from build123d import *

# Parameters (mm, degrees)
SKETCH1_W           = 55
SKETCH1_H           = 80
BOSS_EXTRUDE1_DEPTH = 10
BOSS_EXTRUDE2_DEPTH = 20
BOSS_EXTRUDE3_DEPTH = 30
FILLET1_START       = -1
FILLET1_DEPTH       = 12


with BuildPart() as part:
    # Sketch1 → Boss-Extrude1 (new body)
    # profile 1 of 11: a face of its own
    with BuildSketch(Plane(origin=(0, 0, 0), x_dir=(1, 0, 0), z_dir=(0, 1, 0))):
        with BuildLine():
            ThreePointArc((-40, 70), (-60, 50), (-40, 30))
            Line((-40, 30), (-40, 40))
            ThreePointArc((-40, 40), (-47.071067812, 57.071067812), (-30, 50))
            Line((-30, 50), (-20, 50))
            ThreePointArc((-20, 50), (-25.857864376, 64.142135624), (-40, 70))
        make_face()
    # profile 2 of 11: a face of its own
    with BuildSketch(Plane(origin=(0, 0, 0), x_dir=(1, 0, 0), z_dir=(0, 1, 0))):
        with BuildLine():
            Line((-40, 40), (-40, 30))
            ThreePointArc((-40, 30), (-25.857864376, 35.857864376), (-20, 50))
            Line((-20, 50), (-30, 50))
            ThreePointArc((-30, 50), (-32.928932188, 42.928932188), (-40, 40))
        make_face()
    # profile 3 of 11: a face of its own
    with BuildSketch(Plane(origin=(0, 0, 0), x_dir=(1, 0, 0), z_dir=(0, 1, 0))):
        with BuildLine():
            ThreePointArc((-40, 70), (-60, 50), (-40, 30))
            Line((-40, 30), (-40, 40))
            ThreePointArc((-40, 40), (-47.071067812, 57.071067812), (-30, 50))
            Line((-30, 50), (-20, 50))
            ThreePointArc((-20, 50), (-25.857864376, 64.142135624), (-40, 70))
        make_face()
    # profile 4 of 11: a face of its own
    with BuildSketch(Plane(origin=(0, 0, 0), x_dir=(1, 0, 0), z_dir=(0, 1, 0))):
        with BuildLine():
            Line((-40, 40), (-40, 30))
            ThreePointArc((-40, 30), (-25.857864376, 35.857864376), (-20, 50))
            Line((-20, 50), (-30, 50))
            ThreePointArc((-30, 50), (-32.928932188, 42.928932188), (-40, 40))
        make_face()
    # profile 5 of 11: a face of its own
    with BuildSketch(Plane(origin=(0, 0, 0), x_dir=(1, 0, 0), z_dir=(0, 1, 0))):
        with BuildLine():
            ThreePointArc((-20, 50), (-25.857864376, 35.857864376), (-40, 30))
            Line((-40, 30), (-27.5, 30))
            Line((-27.5, 30), (27.5, 30))
            Line((27.5, 30), (40, 30))
            ThreePointArc((40, 30), (25.857864376, 35.857864376), (20, 50))
            Line((20, 50), (-20, 50))
        make_face()
    # profile 6 of 11: a face of its own
    with BuildSketch(Plane(origin=(0, 0, 0), x_dir=(1, 0, 0), z_dir=(0, 1, 0))):
        with BuildLine():
            ThreePointArc((60, 50), (54.142135624, 64.142135624), (40, 70))
            ThreePointArc((40, 70), (25.857864376, 64.142135624), (20, 50))
            Line((20, 50), (30, 50))
            ThreePointArc((30, 50), (40, 60), (50, 50))
            ThreePointArc((50, 50), (47.071067812, 42.928932188), (40, 40))
            Line((40, 40), (40, 30))
            ThreePointArc((40, 30), (54.142135624, 35.857864376), (60, 50))
        make_face()
    # profile 7 of 11: a face of its own
    with BuildSketch(Plane(origin=(0, 0, 0), x_dir=(1, 0, 0), z_dir=(0, 1, 0))):
        with BuildLine():
            Line((30, 50), (20, 50))
            ThreePointArc((20, 50), (25.857864376, 35.857864376), (40, 30))
            Line((40, 30), (40, 40))
            ThreePointArc((40, 40), (32.928932188, 42.928932188), (30, 50))
        make_face()
    # profile 8 of 11: a face of its own
    with BuildSketch(Plane(origin=(0, 0, 0), x_dir=(1, 0, 0), z_dir=(0, 1, 0))):
        with BuildLine():
            ThreePointArc((60, 50), (54.142135624, 64.142135624), (40, 70))
            ThreePointArc((40, 70), (25.857864376, 64.142135624), (20, 50))
            Line((20, 50), (30, 50))
            ThreePointArc((30, 50), (40, 60), (50, 50))
            ThreePointArc((50, 50), (47.071067812, 42.928932188), (40, 40))
            Line((40, 40), (40, 30))
            ThreePointArc((40, 30), (54.142135624, 35.857864376), (60, 50))
        make_face()
    # profile 9 of 11: a face of its own
    with BuildSketch(Plane(origin=(0, 0, 0), x_dir=(1, 0, 0), z_dir=(0, 1, 0))):
        with BuildLine():
            Line((30, 50), (20, 50))
            ThreePointArc((20, 50), (25.857864376, 35.857864376), (40, 30))
            Line((40, 30), (40, 40))
            ThreePointArc((40, 40), (32.928932188, 42.928932188), (30, 50))
        make_face()
    # profile 10 of 11: a face of its own
    with BuildSketch(Plane(origin=(0, 0, 0), x_dir=(1, 0, 0), z_dir=(0, 1, 0))):
        with Locations((0, -10)):
            Rectangle(SKETCH1_W, SKETCH1_H)
        with BuildLine():
            ThreePointArc((-7.5, -36.09420366), (-17.5, -26.09420366), (-7.5, -16.09420366))
            Line((-7.5, -16.09420366), (7.5, -16.09420366))
            ThreePointArc((7.5, -16.09420366), (17.5, -26.09420366), (7.5, -36.09420366))
            Line((7.5, -36.09420366), (-7.5, -36.09420366))
        make_face(mode=Mode.SUBTRACT)
    # profile 11 of 11: a face of its own
    with BuildSketch(Plane(origin=(0, 0, 0), x_dir=(1, 0, 0), z_dir=(0, 1, 0))):
        with BuildLine():
            Line((40, 70), (-40, 70))
            ThreePointArc((-40, 70), (-25.857864376, 64.142135624), (-20, 50))
            Line((-20, 50), (20, 50))
            ThreePointArc((20, 50), (25.857864376, 64.142135624), (40, 70))
        make_face()
    extrude(amount=BOSS_EXTRUDE1_DEPTH)

    # Sketch2 → Boss-Extrude2 (add)
    with BuildSketch(Plane(origin=(0, 10, 0), x_dir=(1, 0, 0), z_dir=(0, 1, 0))):
        with BuildLine():
            ThreePointArc((40, 30), (30, 32.679491924), (22.679491924, 40))
            Line((22.679491924, 40), (-22.679491924, 40))
            ThreePointArc((-22.679491924, 40), (-30, 32.679491924), (-40, 30))
            Line((-40, 30), (-27.5, 30))
            Line((-27.5, 30), (27.5, 30))
            Line((27.5, 30), (40, 30))
        make_face()
        with BuildLine():
            ThreePointArc((50, 50), (47.071067812, 42.928932188), (40, 40))
            Line((40, 40), (22.679491924, 40))
            ThreePointArc((22.679491924, 40), (30, 32.679491924), (40, 30))
            ThreePointArc((40, 30), (54.142135624, 35.857864376), (60, 50))
            ThreePointArc((60, 50), (54.142135624, 64.142135624), (40, 70))
            ThreePointArc((40, 70), (30, 67.320508076), (22.679491924, 60))
            Line((22.679491924, 60), (40, 60))
            ThreePointArc((40, 60), (47.071067812, 57.071067812), (50, 50))
        make_face()
        with BuildLine():
            Line((22.679491924, 40), (40, 40))
            ThreePointArc((40, 40), (30, 50), (40, 60))
            Line((40, 60), (22.679491924, 60))
            ThreePointArc((22.679491924, 60), (20, 50), (22.679491924, 40))
        make_face()
        with BuildLine():
            ThreePointArc((50, 50), (47.071067812, 42.928932188), (40, 40))
            Line((40, 40), (22.679491924, 40))
            ThreePointArc((22.679491924, 40), (30, 32.679491924), (40, 30))
            ThreePointArc((40, 30), (54.142135624, 35.857864376), (60, 50))
            ThreePointArc((60, 50), (54.142135624, 64.142135624), (40, 70))
            ThreePointArc((40, 70), (30, 67.320508076), (22.679491924, 60))
            Line((22.679491924, 60), (40, 60))
            ThreePointArc((40, 60), (47.071067812, 57.071067812), (50, 50))
        make_face()
        with BuildLine():
            ThreePointArc((-40, 30), (-30, 32.679491924), (-22.679491924, 40))
            Line((-22.679491924, 40), (-40, 40))
            ThreePointArc((-40, 40), (-50, 50), (-40, 60))
            Line((-40, 60), (-22.679491924, 60))
            ThreePointArc((-22.679491924, 60), (-30, 67.320508076), (-40, 70))
            ThreePointArc((-40, 70), (-60, 50), (-40, 30))
        make_face()
        with BuildLine():
            Line((-40, 40), (-22.679491924, 40))
            ThreePointArc((-22.679491924, 40), (-20.681483474, 44.823619098), (-20, 50))
            ThreePointArc((-20, 50), (-20.681483474, 55.176380902), (-22.679491924, 60))
            Line((-22.679491924, 60), (-40, 60))
            ThreePointArc((-40, 60), (-32.928932188, 57.071067812), (-30, 50))
            ThreePointArc((-30, 50), (-32.928932188, 42.928932188), (-40, 40))
        make_face()
        with BuildLine():
            ThreePointArc((-40, 30), (-30, 32.679491924), (-22.679491924, 40))
            Line((-22.679491924, 40), (-40, 40))
            ThreePointArc((-40, 40), (-50, 50), (-40, 60))
            Line((-40, 60), (-22.679491924, 60))
            ThreePointArc((-22.679491924, 60), (-30, 67.320508076), (-40, 70))
            ThreePointArc((-40, 70), (-60, 50), (-40, 30))
        make_face()
    extrude(amount=BOSS_EXTRUDE2_DEPTH)

    # Sketch2_3 → Boss-Extrude3 (add)
    with BuildSketch(Plane(origin=(0, 10, 0), x_dir=(1, 0, 0), z_dir=(0, 1, 0))):
        with BuildLine():
            ThreePointArc((-40, 30), (-30, 32.679491924), (-22.679491924, 40))
            Line((-22.679491924, 40), (-40, 40))
            ThreePointArc((-40, 40), (-50, 50), (-40, 60))
            Line((-40, 60), (-22.679491924, 60))
            ThreePointArc((-22.679491924, 60), (-30, 67.320508076), (-40, 70))
            ThreePointArc((-40, 70), (-60, 50), (-40, 30))
        make_face()
        with BuildLine():
            ThreePointArc((-40, 30), (-30, 32.679491924), (-22.679491924, 40))
            Line((-22.679491924, 40), (-40, 40))
            ThreePointArc((-40, 40), (-50, 50), (-40, 60))
            Line((-40, 60), (-22.679491924, 60))
            ThreePointArc((-22.679491924, 60), (-30, 67.320508076), (-40, 70))
            ThreePointArc((-40, 70), (-60, 50), (-40, 30))
        make_face()
        with BuildLine():
            Line((-40, 40), (-22.679491924, 40))
            ThreePointArc((-22.679491924, 40), (-20.681483474, 44.823619098), (-20, 50))
            ThreePointArc((-20, 50), (-20.681483474, 55.176380902), (-22.679491924, 60))
            Line((-22.679491924, 60), (-40, 60))
            ThreePointArc((-40, 60), (-32.928932188, 57.071067812), (-30, 50))
            ThreePointArc((-30, 50), (-32.928932188, 42.928932188), (-40, 40))
        make_face()
    extrude(amount=BOSS_EXTRUDE3_DEPTH)

    # Fillet1: read off the stored shape, not the designer's step
    # Fillet1 outline → Fillet1 (cut)
    with BuildSketch(Plane(origin=(0, 0, 0), x_dir=(1, 0, 0), z_dir=(0, 1, 0)).offset(FILLET1_START)):
        with BuildLine():
            ThreePointArc((27.5, -40), (24.571067812, -47.071067812), (17.5, -50))
            Line((17.5, -50), (27.5, -50))
            Line((27.5, -50), (27.5, -40))
        make_face()
        with BuildLine():
            ThreePointArc((-17.5, -50), (-24.571067812, -47.071067812), (-27.5, -40))
            Line((-27.5, -40), (-27.5, -50))
            Line((-27.5, -50), (-17.5, -50))
        make_face()
    extrude(amount=FILLET1_DEPTH, mode=Mode.SUBTRACT)


solid = part.part
CAD build for the part. Positions are in the model's coordinates, mm. A direction names the side the tool comes from. Give positions to 0.01 mm unless a question says otherwise; leave off trailing zeros. Loops run counter-clockwise (first coordinate to the right, second up) from the corner with the lowest first, then second, coordinate; pieces in that order, holes last. Notation, with made-up numbers: M 85,25.25 L 95,25.25 A18 cw 95,41.25 Z; hole C 15.25,30 d5. An arc over 180 degrees is marked long. Write each question's results on one line, items separated by ' | '.
Q1. Band-saw the part on D-D on x = -52. Write the cut outline in (y, z), and give its area (3 significant figures).
Geometry check:
outline: M 0,-66 L 40,-66 L 40,-34 L 0,-34 Z | area: 1,280 mm²
Q2. Probe probe 1 along X at (y, z) = (13, -50); probe 2 along Z at (x, y) = (-40, 23.5); probe 3 along X at (y, z) = (22.5, -52). List the from-to ranges inside material, lowest first.
Geometry check:
probe 1: x = -60 to -50, -30 to -20, 20 to 30, 50 to 60 | probe 2: z = -70 to -60, -40 to -30 | probe 3: x = -59.9 to -49.8, -30.2 to -20.1, 20.1 to 30.2, 49.8 to 59.9
Q3. Which spindle directions (+Z, -Z, +X, -X, +Y, -Y) get a long thin tool onto all of the face, cutting with end or side? Do faces 5 (the face through (0, 10, 9)), 6 (the face through (27.5, 5, 5)), 7 (the face through (0, 5, 36.094)), 8 (the face through (-49, 40, -55)), 9 (the face through (0, 5, 50)). Say none if no direction does.
Geometry check:
face 5: +Z, +X, -X, +Y | face 6: +Z, +X, +Y, -Y | face 7: +Y, -Y | face 8: +Z, -Z, +X, -X, +Y | face 9: +Z, +X, -X, +Y, -Y
Q4. Flat gauge pins, fed straight in: P1, Ø11, axis at y = 6, z = -9.5, coming from the -X side; P2, Ø6, axis at x = 25, y = 29, coming from the +Z side; P3, Ø16, axis at x = 6, y = 24.5, coming from the -Z side. Where does each tip first touch, or does it go through?
Geometry check:
P1: stops at x = -27.5 | P2: stops at z = -30 | P3: stops at z = -40
Q5. Band-saw the part on A-A on y = 5.5. Write the cut outline in (x, z).
Geometry check:
outline: M -40,-70 L 40,-70 A20 ccw 40,-30 L 27.5,-30 L 27.5,40 A10 ccw 17.5,50 L -17.5,50 A10 ccw -27.5,40 L -27.5,-30 L -40,-30 A20 ccw Z; hole C -40,-50 d20; hole M -7.5,16.09 L 7.5,16.09 A10 ccw 7.5,36.09 L -7.5,36.09 A10 ccw Z; hole C 40,-50 d20
Q6. Mould opens along Z. For faces 1 (the face through (-17.498, 4.93, 26.314)), 2 (the face through (-27.5, 5, 5)), 3 (the face through (1, 5, -70)), 4 (the face through (24.65, 4.93, 46.99)) say: pulls with the +Z half, pulls with the -Z half, needs draft (parallel to the pull), parting line crosses it, or undercut.
Geometry check:
face 1: undercut | face 2: needs draft | face 3: pulls with the -Z half | face 4: pulls with the +Z half
Q7. Band-saw the part on B-B on y = 23. Write the cut outline in (x, z).
Geometry check:
outline: M -40,-30 A20 ccw long -22.68,-40 L 22.68,-40 A20 ccw long 40,-30 Z; hole C -40,-50 d20; hole C 40,-50 d20
